Model file for the job. Use its own axes, mm. A direction names the side the tool comes from. Coordinates: 2 decimals unless noted, no trailing zeros. Write each loop counter-clockwise with the first axis right and the second up, starting at its lowest first coordinate (ties: lowest second). Pieces come first, ordered by that corner, then holes. Notation, with made-up numbers: M -14,8 L 43,8 A13 cw 43,24 Z; hole C 42,-37.75 d10. An arc over 180 degrees is marked long. One line per question, with ' | ' between items. Start each with the question number.
(1) Cut at A-A (x = 0). Write the cut outline in (y, z), plus the area to 3 significant figures.
(2) Wall check: probe 1 along Y at (x, z) = (-64.5, 1.1); probe 2 along Y at (x, z) = (-10, 0.95); probe 3 along X at (y, z) = (-72, 4.25). Give the ranges that are in metal, low to high.
(3) Cut at D-D (x = -103). Write the cut outline in (y, z), plus the area to 3 significant figures.
(4) Two-plate mould, pull along X, no slides. Class faces 4 (the face through (-45, 48, 3)), 5 (the face through (25, 2, 5.2)), 6 (the face through (-37.482, -92.871, 2.564)): +X half, -X half, draft (parallel to the pull), parting line (faces both ways), or undercut.
(5) Flat gauge pins, fed straight in: pin 1 Ø2.5 at (x, y) = (64.5, -71.5) entering from -Z; pin 2 Ø2 at (y, z) = (-26.5, 3) entering from +X; pin 3 Ø2.5 at (y, z) = (-47.5, 1.5) entering from -X; pin 4 Ø2.5 at (y, z) = (-40, 3.5) entering from +X. Where does each tip first touch, or does it go through?
(6) Tool access for faces 1 (the face through (-2, -5, 2.6)), 2 (the face through (71.999, 106.685, 2.564)), 3 (the face through (0, 31, 3)): list every direction of +Z, -Z, +X, -X, +Y, -Y with a clear straight run to the whole face (end or side of a thin tool).
(7) Cut at B-B (z = 1.75). Write the cut outline in (x, y), plus the area to 3 significant figures.
(8) Cut at C-C (y = 0). Write the cut outline in (x, z).
Autodesk Fusion 360 part; units mm, degrees
sketch "Sketch1" plane through (0, 0, 0) normal (0, 0, 1) x (1, 0, 0)
  circle A0 centre (-64.5, 71.5) radius 2.25
  circle A1 centre (64.5, 71.5) radius 2.25
  circle A2 centre (-64.5, -71.5) radius 2.25
  circle A3 centre (64.5, -71.5) radius 2.25
  line L0 (20, 100) -> (-20, 100)
  line L1 (-20, -100) -> (20, -100)
  arc A4 (-20, 100) -> (-45, 75) centre (-20, 75) ccw
  arc A5 (45, 75) -> (20, 100) centre (20, 75) ccw
  arc A6 (20, -100) -> (45, -75) centre (20, -75) ccw
  arc A7 (-45, -75) -> (-20, -100) centre (-20, -75) ccw
  line L2 (45, 20) -> (-45, -20) construction
  circle A8 centre (0, 0) radius 5
  line L3 (64.5, 71.5) -> (-64.5, 71.5) construction
  line L4 (-64.5, 71.5) -> (-64.5, -71.5) construction
  line L5 (-64.5, -71.5) -> (64.5, -71.5) construction
  line L6 (64.5, -71.5) -> (64.5, 71.5) construction
  line L7 (64.5, 71.5) -> (-64.5, -71.5) construction
  line L8 (-64.5, 71.5) -> (64.5, -71.5) construction
  line L9 (45, 20) -> (23.6854, 20)
  line L10 (-23.6854, 20) -> (-45, 20)
  line L11 (-45, 75) -> (-45, 20)
  line L12 (-45, -20) -> (-45, -75)
  arc A9 (-23.6854, -20) -> (23.6854, -20) centre (0, 0) ccw
  arc A10 (23.6854, 20) -> (-23.6854, 20) centre (0, 0) ccw
  line L13 (45, -75) -> (45, -20)
  line L14 (45, 20) -> (45, 75)
  line L15 (-45, 20) -> (4.5691, -2.0307) construction
  line L16 (28.3282, -12.5903) -> (45, -20) construction
  line L17 (-45, -20) -> (-23.6854, -20)
  line L18 (23.6854, -20) -> (45, -20)
  line L19 (91.0962, 100.9826) -> (104.4615, 88.9257) construction
  line L20 (91.0962, 100.9826) -> (77.7308, 113.0394) construction
  line L21 (104.4615, 88.9257) -> (92.8349, 76.0373)
  line L22 (77.7308, 113.0394) -> (66.1042, 100.151)
  arc A11 (104.4615, 88.9257) -> (77.7308, 113.0394) centre (91.0962, 100.9826) ccw
  arc A12 (66.1042, 100.151) -> (92.8349, 76.0373) centre (0, 0) ccw
  dimension "d14" = 4.5
  dimension "d15" = 4.5
  dimension "d16" = 4.5
  dimension "d17" = 4.5
  dimension "d20" = 240
  dimension "d21" = 25
  dimension "d23" = 40
  dimension "d24" = 10
  dimension "d25" = 62
  dimension "d26" = 129
  dimension "d27" = 143
  dimension "d29" = 36
  dimension "d33" = 45
  dimension "d34" = 100
  dimension "d35" = 100
  dimension "d36" = 149.4615
  dimension "d37" = 132.054
  dimension "d38" = 213.0394
  dimension "d39" = 18.2443
  dimension "d40" = 18
extrude "Extrude1" add sketch "Sketch1" along normal blind 5.2
sketch "Sketch4" plane through (0, 0, 5.2) normal (0, 0, 1) x (-1, 0, 0)
  circle A0 centre (-64.5, 71.5) radius 2.25
  circle A1 centre (64.5, 71.5) radius 2.25
  line L0 (-45, -20) -> (-23.6854, -20)
  arc A2 (-23.6854, -20) -> (23.6854, -20) centre (0, 0) ccw
  line L1 (23.6854, -20) -> (45, -20)
  line L2 (45, -20) -> (45, -75)
  arc A3 (20, -100) -> (45, -75) centre (20, -75) ccw
  line L3 (20, -100) -> (-20, -100)
  arc A4 (-45, -75) -> (-20, -100) centre (-20, -75) ccw
  line L4 (-45, -75) -> (-45, -20)
  circle A5 centre (64.5, -71.5) radius 2.25
  circle A6 centre (0, 0) radius 5
  line L5 (45, 75) -> (45, 20)
  line L6 (45, 20) -> (23.6854, 20)
  arc A7 (23.6854, 20) -> (-23.6854, 20) centre (0, 0) ccw
  line L7 (-23.6854, 20) -> (-45, 20)
  line L8 (-45, 20) -> (-45, 75)
  arc A8 (-20, 100) -> (-45, 75) centre (-20, 75) ccw
  line L9 (-20, 100) -> (20, 100)
  arc A9 (45, 75) -> (20, 100) centre (20, 75) ccw
  circle A10 centre (-64.5, -71.5) radius 2.25
  arc A11 (-104.4615, -88.9257) -> (-77.7308, -113.0394) centre (-91.0962, -100.9826) ccw
  line L10 (-77.7308, -113.0394) -> (-66.1042, -100.151)
  arc A12 (-66.1042, -100.151) -> (-92.8349, -76.0373) centre (0, 0) ccw
  line L11 (-92.8349, -76.0373) -> (-104.4615, -88.9257)
  circle A13 centre (0, 0) radius 10
  dimension "d30" = 20
extrude "Extrude3" cut sketch "Sketch4" against normal blind 2.6 contours A13
equation "d31 = ( -5.2 / 2 ) * 1 mm"
Filled in:
1) outline: M -120,0 L -100,0 L -100,5.2 L -120,5.2 Z; M -31,0 L -5,0 L -5,2.6 L -10,2.6 L -10,5.2 L -31,5.2 Z; M 5,0 L 31,0 L 31,5.2 L 10,5.2 L 10,2.6 L 5,2.6 Z; M 100,0 L 120,0 L 120,5.2 L 100,5.2 Z | area: 452 mm²
2) probe 1: -101.19 to -73.75, -69.25 to 69.25, 73.75 to 101.19 | probe 2: -119.58 to -100, -29.34 to 29.34, 100 to 119.58 | probe 3: -96 to -66.69, -62.31 to -45, 45 to 62.31, 66.69 to 96
3) outline: M -61.57,0 L 61.57,0 L 61.57,5.2 L -61.57,5.2 Z | area: 640 mm²
4) face 4: undercut | face 5: draft | face 6: undercut
5) pin 1: through | pin 2: x = 117.26 | pin 3: x = -110.73 | pin 4: x = 113.57
6) face 1: +Z | face 2: +Z, -Z, +Y | face 3: +Z, -Z
7) outline: M 66.1,100.15 A120 ccw long 92.83,76.04 L 104.46,88.93 A18 ccw 77.73,113.04 Z; hole C -64.5,-71.5 d4.5; hole C -64.5,71.5 d4.5; hole M -45,-75 A25 ccw -20,-100 L 20,-100 A25 ccw 45,-75 L 45,-20 L 23.69,-20 A31 cw -23.69,-20 L -45,-20 Z; hole M -45,20 L -23.69,20 A31 cw 23.69,20 L 45,20 L 45,75 A25 ccw 20,100 L -20,100 A25 ccw -45,75 Z; hole C 0,0 d10; hole C 64.5,-71.5 d4.5; hole C 64.5,71.5 d4.5 | area: 33,100 mm²
8) outline: M -120,0 L -5,0 L -5,2.6 L -10,2.6 L -10,5.2 L -120,5.2 Z; M 5,0 L 120,0 L 120,5.2 L 10,5.2 L 10,2.6 L 5,2.6 Z
